from build123d import *

# Parameters (mm, degrees)
SKETCH1_W           = 304.8
SKETCH1_H           = 228.6
BOSS_EXTRUDE1_DEPTH = 12.7
SKETCH2_R           = 4.7625
CUT_EXTRUDE1_DEPTH  = 12.7
SKETCH7_W           = 112.268
SKETCH7_H           = 12.7
CUT_EXTRUDE2_DEPTH  = 12.7
SKETCH8_W           = 12.7
SKETCH8_H           = 228.6
SKETCH8_W_2         = 3.175
BOSS_EXTRUDE2_DEPTH = 12.7


with BuildPart() as part:
    # Sketch1 → Boss-Extrude1 (new body)
    with BuildSketch(Plane.XY):
        with Locations((152.4, 114.3)):
            Rectangle(SKETCH1_W, SKETCH1_H)
    extrude(amount=BOSS_EXTRUDE1_DEPTH)

    # Sketch2 → Cut-Extrude1 (cut)
    with BuildSketch(Plane.XY.offset(12.7)):
        with Locations((91.44, 114.3)):
            Circle(SKETCH2_R)
    extrude(amount=-CUT_EXTRUDE1_DEPTH, mode=Mode.SUBTRACT)

    # Sketch7 → Cut-Extrude2 (cut)
    with BuildSketch(Plane.XY.offset(12.7)):
        with Locations((70.358, 222.25)):
            Rectangle(SKETCH7_W, SKETCH7_H)
        with Locations((234.442, 222.25)):
            Rectangle(SKETCH7_W, SKETCH7_H)
        with Locations((70.358, 196.85)):
            Rectangle(SKETCH7_W, SKETCH7_H)
        with Locations((234.442, 196.85)):
            Rectangle(SKETCH7_W, SKETCH7_H)
    extrude(amount=-CUT_EXTRUDE2_DEPTH, mode=Mode.SUBTRACT)

    # Sketch8 → Boss-Extrude2 (add)
    with BuildSketch(Plane.XY.offset(12.7)):
        with Locations((-6.35, 114.3)):
            Rectangle(SKETCH8_W, SKETCH8_H)
        with Locations((306.3875, 114.3)):
            Rectangle(SKETCH8_W_2, SKETCH8_H)
    extrude(amount=-BOSS_EXTRUDE2_DEPTH)


solid = part.part
Verification items for the finished model (mm, model axes). A direction names the side the tool comes from. Coordinates: 2 decimals unless noted, no trailing zeros. Loops run counter-clockwise (first coordinate to the right, second up) from the corner with the lowest first, then second, coordinate; pieces in that order, holes last. Notation, with made-up numbers: (71.25, -33.5) -> (116.25, -33.5) arc R15 cw to (116.25, -15.5) -> close; hole circle Ø8 at (75.5, -32.5). An arc over 180 degrees is marked (long way). Write each question's results on one line, items separated by ' | '.
Item 1: Section check D-D, the plane x = 91.44. Enter the section's corners in (y, z).
Found:
outline: (0, 0) -> (109.54, 0) -> (109.54, 12.7) -> (0, 12.7) -> close; (119.06, 0) -> (190.5, 0) -> (190.5, 12.7) -> (119.06, 12.7) -> close; (203.2, 0) -> (215.9, 0) -> (215.9, 12.7) -> (203.2, 12.7) -> close
Item 2: Material ranges on L1, parallel to X at y = 200.5, z = 2.5 (3 decimals); L2, parallel to Y at x = 91.44, z = 3; L3, parallel to Y at x = 267, z = 4.25, recorded low to high.
Found:
L1: x = -12.7 to 14.224, 126.492 to 178.308, 290.576 to 307.975 | L2: y = 0 to 109.54, 119.06 to 190.5, 203.2 to 215.9 | L3: y = 0 to 190.5, 203.2 to 215.9
Item 3: Tool access check on faces 1 (the face through (145, 91, 0)), 2 (the face through (234, 203.2, 6)), 3 (the face through (178.308, 222, 6)). Record the directions out of +Z, -Z, +X, -X, +Y, -Y that give a thin tool (end or side, any length) a straight path to the whole face; none if there is none.
Found:
face 1: -Z, +X, -X, +Y, -Y | face 2: +Z, -Z | face 3: +Z, -Z, +Y
Item 4: Gauge pin test, flat ends, axial feed: pin 1 (5.5 mm diameter, centred on x = 91.44, y = 114.3, fed in from -Z) (3 decimals); pin 2 (6.5 mm diameter, centred on x = 230, z = 8.5, fed in from +Y). Record the tip position at first contact, or that the pin passes through.
Found:
pin 1: passes through | pin 2: stops at y = 215.9
Item 5: Section check C-C, the plane y = 114.3. Enter the section's corners in (x, z) (1 decimal).
Found:
outline: (-12.7, 0) -> (86.7, 0) -> (86.7, 12.7) -> (-12.7, 12.7) -> close; (96.2, 0) -> (308, 0) -> (308, 12.7) -> (96.2, 12.7) -> close
Item 6: Section check A-A, the plane x = 19. Enter the section's corners in (y, z).
Found:
outline: (0, 0) -> (190.5, 0) -> (190.5, 12.7) -> (0, 12.7) -> close; (203.2, 0) -> (215.9, 0) -> (215.9, 12.7) -> (203.2, 12.7) -> close
Item 7: Section check B-B, the plane z = 10.75. Enter the section's corners in (x, y) (1 decimal), plus the area to 3 significant figures.
Found:
outline: (-12.7, 0) -> (308, 0) -> (308, 228.6) -> (290.6, 228.6) -> (290.6, 215.9) -> (178.3, 215.9) -> (178.3, 228.6) -> (126.5, 228.6) -> (126.5, 215.9) -> (14.2, 215.9) -> (14.2, 228.6) -> (-12.7, 228.6) -> close; hole (14.2, 190.5) -> (126.5, 190.5) -> (126.5, 203.2) -> (14.2, 203.2) -> close; hole circle Ø9.5 at (91.4, 114.3); hole (178.3, 190.5) -> (290.6, 190.5) -> (290.6, 203.2) -> (178.3, 203.2) -> close | area: 67,500 mm2
Item 8: Mould release check, pull along X, two halves, no side actions. Record for faces 4 (the face through (145, 91, 12.7)), 5 (the face through (-12.7, 113, 6)), 6 (the face through (178.308, 197, 6)): +X half, -X half, draft (parallel to the pull), parting line (faces both ways), or undercut.
Found:
face 4: draft | face 5: -X half | face 6: undercut
